Input: part model. Units: mm. Frame: model coordinates. A direction names the side the tool comes from. Give positions to 0.01 mm unless a question says otherwise; leave off trailing zeros. Write each loop counter-clockwise with the first axis right and the second up, starting at its lowest first coordinate (ties: lowest second). Pieces come first, ordered by that corner, then holes. Notation, with made-up numbers: (89.25, 40.25) - (142.25, 40.25) arc R14 cw to (142.25, 66.25) - close; hole circle Ø1 at (1, -2.5). An arc over 180 degrees is marked (long way). Answer as CSV lines item,"result". Start each with the question number.
from build123d import *

# Parameters (mm, degrees)
SALIENTE_EXTRUIR1_DEPTH = 25
NERVIO1_REACH           = 90.369
CROQUIS3_WALL_W         = 202.590813764
CROQUIS3_WALL_H         = 2
REDONDEO1_R             = 2
CROQUIS4_R              = 11.05
CROQUIS4_R_2            = 2
CORTAR_EXTRUIR1_DEPTH   = 76
CHAFL_N1_SIZE           = 5
CORTAR_EXTRUIR2_DEPTH   = 76.119904153
CROQUIS6_R              = 2
CORTAR_EXTRUIR3_DEPTH   = 76.119904153


with BuildPart() as part:
    # Croquis2 → Saliente-Extruir1 (new, symmetric)
    with BuildSketch(Plane(origin=(0, 0, 0), x_dir=(0, 0, -1), z_dir=(1, 0, 0))):
        Polygon((0, 0), (-53, 0), (-53, 3), (-3, 3), (-3, 50), (0, 50), align=None)
    extrude(amount=SALIENTE_EXTRUIR1_DEPTH, both=True)

    # Croquis3 wall → Nervio1 (add, up to next)
    with BuildSketch(Plane(origin=(25, 13, 9.5), x_dir=(0, 0.838443616301, -0.544988350595), z_dir=(0, 0.544988350595, 0.838443616301)), mode=Mode.PRIVATE) as nervio1_sk1:
        with Locations((0, 1)):
            Rectangle(CROQUIS3_WALL_W, CROQUIS3_WALL_H)
    nervio1_tool1 = extrude(nervio1_sk1.sketch, amount=-NERVIO1_REACH, mode=Mode.PRIVATE) - part.part
    nervio1 = nervio1_tool1.solids().sort_by_distance((25, 13, 9.5))[0]
    add(nervio1)

    # Simetría1: Nervio1 across plane
    add(nervio1.mirror(Plane(origin=(0, 0, 0), x_dir=(0, 0, 1), z_dir=(1, 0, 0))))

    # Redondeo1
    redondeo1_edges = [part.edges().sort_by_distance(p)[0] for p in [
        (0, 0, 0),
        (0, 3, 3),
    ]]
    fillet(redondeo1_edges, radius=REDONDEO1_R)

    # Croquis4 → Cortar-Extruir1 (cut, through all)
    with BuildSketch(Plane.XY.offset(3)):
        with Locations((0, 29)):
            Circle(CROQUIS4_R)
        with Locations((-15.5, 44.5)):
            Circle(CROQUIS4_R_2)
        with Locations(Location((15.5, 44.5, 0), (0, 0, 180))):
            Circle(CROQUIS4_R_2)
        with Locations(Location((-15.5, 13.5, 0), (0, 0, 180))):
            Circle(CROQUIS4_R_2)
        with Locations((15.5, 13.5)):
            Circle(CROQUIS4_R_2)
    extrude(amount=-CORTAR_EXTRUIR1_DEPTH, mode=Mode.SUBTRACT)

    # Chaflán1
    chafl_n1_edges = [part.edges().sort_by_distance(p)[0] for p in [
        (25, 1.5, 53),
        (-25, 1.5, 53),
        (-25, 50, 1.5),
        (25, 50, 1.5),
    ]]
    chamfer(chafl_n1_edges, length=CHAFL_N1_SIZE)

    # Croquis5 → Cortar-Extruir2 (cut, through all)
    with BuildSketch(Plane(origin=(0, 3, 0), x_dir=(1, 0, 0), z_dir=(0, 1, 0))):
        with BuildLine():
            Line((-13.85, -13), (-13.85, -43))
            ThreePointArc((-13.85, -43), (-16, -45.15), (-18.15, -43))
            Line((-18.15, -43), (-18.15, -13))
            ThreePointArc((-18.15, -13), (-16, -10.85), (-13.85, -13))
        make_face()
        with BuildLine():
            Line((13.85, -13), (13.85, -43))
            ThreePointArc((13.85, -43), (16, -45.15), (18.15, -43))
            Line((18.15, -43), (18.15, -13))
            ThreePointArc((18.15, -13), (16, -10.85), (13.85, -13))
        make_face()
    extrude(amount=-CORTAR_EXTRUIR2_DEPTH, mode=Mode.SUBTRACT)

    # Croquis6 → Cortar-Extruir3 (cut, through all)
    with BuildSketch(Plane(origin=(0, 3, 0), x_dir=(1, 0, 0), z_dir=(0, 1, 0))):
        with Locations(Location((0, -13, 0), (0, 0, 270))):
            Circle(CROQUIS6_R)
        with Locations(Location((0, -43, 0), (0, 0, 90))):
            Circle(CROQUIS6_R)
    extrude(amount=-CORTAR_EXTRUIR3_DEPTH, mode=Mode.SUBTRACT)


solid = part.part
1) Reachability of faces 5 (the flat face through (18.15, 2, 28)), 6 (the flat face through (-22, 1, 51)), 7 (the flat face through (0, 3, 29)) from +Z, -Z, +X, -X, +Y, -Y: full face, straight path, thin tool, end or side. Return the list, or none.
2) Pull-direction query (X, two-part tool) for faces 1 (the flat face through (23, 1, 50)), 2 (the flat face through (-23, 9, 8)), 3 (the flat face through (23.99, 12.86, 9.59)), 4 (the cylindrical face through (-16.05, 1.52, 10.85)); classes: +X half, -X half, draft (parallel to the pull), parting line (faces both ways), or undercut.
3) Cut plane A-A on x = 0. Output: boundary loops of the cut face in (y, z).
4) Cut plane D-D on x = -8. Output: boundary loops of the cut face in (y, z), and give its area (3 significant figures).
5) Material intervals for line 1 (X direction, y = 2.3, z = 13); line 2 (Y direction, x = -15.5, z = 1.15), sorted ascending. Write a range as from..to.
6) Cut plane B-B on z = 23. Output: boundary loops of the cut face in (x, y).
7) Cut plane C-C on y = 32. Output: boundary loops of the cut face in (x, z).
8) Contact query for flat-ended pins moving along their axis: P1, Ø4, axis at x = -15, z = 13.5, coming from the -Y side; P2, Ø3, axis at x = 0, z = 43, coming from the -Y side; P3, Ø6, axis at x = 9, z = 6.5, coming from the +Y side; P4, Ø3, axis at x = -9.5, z = 42.5, coming from the +Y side. Output: stop coordinate, or through.
Numbers:
1,face 5,"+Y, -Y"
1,face 6,"+Z, -X, +Y, -Y"
1,face 7,"+Z, +Y"
2,face 1,"+X half"
2,face 2,"undercut"
2,face 3,"draft"
2,face 4,"undercut"
3,outline,"(0, 2) arc R2 ccw to (2, 0) - (17.95, 0) - (17.95, 3) - (5, 3) arc R2 cw to (3, 5) - (3, 11) - (0, 11) - close; (0, 15) - (3, 15) - (3, 41) - (0, 41) - close; (0, 45) - (3, 45) - (3, 53) - (0, 53) - close; (40.05, 0) - (50, 0) - (50, 3) - (40.05, 3) - close"
4,outline,"(0, 2) arc R2 ccw to (2, 0) - (21.38, 0) - (21.38, 3) - (5, 3) arc R2 cw to (3, 5) - (3, 53) - (0, 53) - close; (36.62, 0) - (50, 0) - (50, 3) - (36.62, 3) - close"
4,area,"254 mm²"
5,line 1,"x = -25..-18.15, -13.85..-2, 2..13.85, 18.15..25"
5,line 2,"y = 0.19..11.5, 15.5..42.5, 46.5..50"
6,outline,"(-25, 0) - (-18.15, 0) - (-18.15, 3) - (-25, 3) - close; (-13.85, 0) - (13.85, 0) - (13.85, 3) - (-13.85, 3) - close; (18.15, 0) - (25, 0) - (25, 3) - (18.15, 3) - close"
7,outline,"(-25, 0) - (-10.63, 0) - (-10.63, 3) - (-25, 3) - close; (10.63, 0) - (25, 0) - (25, 3) - (10.63, 3) - close"
8,P1,"stops at y = 0"
8,P2,"passes through"
8,P3,"stops at y = 3.68"
8,P4,"stops at y = 3"
